from build123d import *

# Parameters (mm, degrees)
SKETCH031_R        = 14.25
SKETCH031_R_2      = 1
PAD007_DEPTH       = 0.3
POCKET_DEPTH       = 80.913406
POLARPATTERN_COUNT = 4


with BuildPart() as part:
    # Sketch031 → Pad007 (new body)
    with BuildSketch(Plane.XY.offset(0.7)):
        Circle(SKETCH031_R)
        Circle(SKETCH031_R_2, mode=Mode.SUBTRACT)
    extrude(amount=PAD007_DEPTH)

    # Sketch → Pocket (cut, through all)
    with BuildSketch(Plane.XY.offset(1)):
        with BuildLine():
            Line((-1.141945, 13.451616), (1.141945, 13.451616))
            ThreePointArc((1.379292, 13.123091), (1.344591, 13.34802), (1.141945, 13.451616))
            Line((1.379292, 13.123091), (0.237348, 9.671475))
            ThreePointArc((-0.237348, 9.671475), (0, 9.5), (0.237348, 9.671475))
            Line((-0.237348, 9.671475), (-1.379292, 13.123091))
            ThreePointArc((-1.141945, 13.451616), (-1.344591, 13.34802), (-1.379292, 13.123091))
        make_face()
        with BuildLine():
            Line((4.333734, 8.756248), (6.081129, 11.782825))
            ThreePointArc((6.422636, 11.874332), (6.232931, 11.899307), (6.081129, 11.782825))
            Line((6.422636, 11.874332), (7.072155, 11.499332))
            ThreePointArc((7.163661, 11.157825), (7.188636, 11.34753), (7.072155, 11.499332))
            Line((7.163661, 11.157825), (5.416266, 8.131248))
            ThreePointArc((5.07476, 8.039741), (5.264464, 8.014766), (5.416266, 8.131248))
            Line((5.07476, 8.039741), (4.42524, 8.414741))
            ThreePointArc((4.333734, 8.756248), (4.308759, 8.566543), (4.42524, 8.414741))
        make_face()
        with BuildLine():
            Line((8.131248, 5.416266), (11.157825, 7.163661))
            ThreePointArc((11.499332, 7.072155), (11.34753, 7.188636), (11.157825, 7.163661))
            Line((11.499332, 7.072155), (11.874332, 6.422636))
            ThreePointArc((11.782825, 6.081129), (11.899307, 6.232931), (11.874332, 6.422636))
            Line((11.782825, 6.081129), (8.756248, 4.333734))
            ThreePointArc((8.414741, 4.42524), (8.566543, 4.308759), (8.756248, 4.333734))
            Line((8.414741, 4.42524), (8.039741, 5.07476))
            ThreePointArc((8.131248, 5.416266), (8.014766, 5.264464), (8.039741, 5.07476))
        make_face()
    pocket = extrude(amount=-POCKET_DEPTH, mode=Mode.SUBTRACT)

    # PolarPattern: Pocket ×4 about axis
    polarpattern_axis = Axis((0, 0, 1), (0, 0, 1))
    for i in range(1, POLARPATTERN_COUNT):
        add(pocket.rotate(polarpattern_axis, i * 360 / POLARPATTERN_COUNT), mode=Mode.SUBTRACT)


solid = part.part
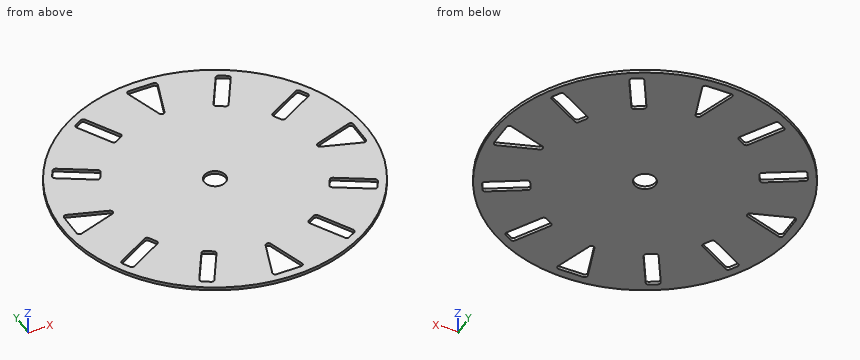
Input: part model. Units: mm. Frame: model coordinates. Give positions to 0.01 mm unless a question says otherwise; leave off trailing zeros. Order: outer loops, then holes, each group sorted by start corner. A loop starts at its lowest first (then second) coordinate and runs counter-clockwise, first axis right, second up. Notation, with made-up numbers: M -31.5,56.25 L -7.5,56.25 A21 ccw -7.5,71.25 Z; hole C 24,48.25 d5. An arc over 180 degrees is marked long. Answer as a JSON object with one key per item and string values.
1. Cut plane B-B, the plane z = 0.9. State how many separate pieces and enclosed holes the cut face has, and give its area (3 significant figures).
Result sheet:
{"separate pieces": "1", "enclosed holes": "13", "area": "569 mm²"}
2. Cut plane A-A, the plane y = -12.5. Output: boundary loops of the cut face in (x, z), and give its area (3 significant figures).
Result sheet:
{"outline": "M -6.84,0.7 L -1.17,0.7 L -1.17,1 L -6.84,1 Z; M 1.17,0.7 L 6.84,0.7 L 6.84,1 L 1.17,1 Z", "area": "3.40 mm²"}
3. Cut plane D-D, the plane x = -3.25. Output: boundary loops of the cut face in (y, z).
Result sheet:
{"outline": "M -13.87,0.7 L 13.87,0.7 L 13.87,1 L -13.87,1 Z"}
4. Ray query, line 1 (Y direction, x = 0, z = 0.85); line 2 (X direction, y = 8.5, z = 0.8); line 3 (Y direction, x = 10.5, z = 0.8). Return the intervals inside material, ascending. Write a range as [from, to].
Result sheet:
{"line 1": "[-14.25, -13.45], [-9.5, -1], [1, 9.5], [13.45, 14.25]", "line 2": "[-11.44, -5.63], [-4.34, 4.34], [5.63, 11.44]", "line 3": "[-9.63, -6.78], [-5.34, -0.51], [0.51, 5.34], [6.78, 9.63]"}
5. Cut plane C-C, the plane x = 3.5. Output: boundary loops of the cut face in (y, z).
Result sheet:
{"outline": "M -13.81,0.7 L 13.81,0.7 L 13.81,1 L -13.81,1 Z"}
